```python
from build123d import *

# Parameters (mm, degrees)
SKETCH1_R           = 47.5
SKETCH1_R_2         = 10.5
SKETCH1_R_3         = 2.7
BOSS_EXTRUDE1_DEPTH = 6
SKETCH2_R           = 12
CUT_EXTRUDE1_DEPTH  = 2
BOSS_EXTRUDE2_START = 3
SKETCH3_R           = 16
SKETCH3_R_2         = 12
BOSS_EXTRUDE2_DEPTH = 3
SKETCH4_R           = 2.7
CUT_EXTRUDE2_DEPTH  = 5


with BuildPart() as part:
    # Sketch1 → Boss-Extrude1 (new body)
    with BuildSketch(Plane.XY):
        Circle(SKETCH1_R)
        Circle(SKETCH1_R_2, mode=Mode.SUBTRACT)
        with Locations((44, 0)):
            Circle(SKETCH1_R_3, mode=Mode.SUBTRACT)
        with Locations((22, -38.105117767)):
            Circle(SKETCH1_R_3, mode=Mode.SUBTRACT)
        with Locations((-22, -38.105117767)):
            Circle(SKETCH1_R_3, mode=Mode.SUBTRACT)
        with Locations((-44, 0)):
            Circle(SKETCH1_R_3, mode=Mode.SUBTRACT)
        with Locations((-22, 38.105117767)):
            Circle(SKETCH1_R_3, mode=Mode.SUBTRACT)
        with Locations((22, 38.105117767)):
            Circle(SKETCH1_R_3, mode=Mode.SUBTRACT)
    extrude(amount=BOSS_EXTRUDE1_DEPTH)

    # Sketch2 → Cut-Extrude1 (cut)
    with BuildSketch(Plane(origin=(0, 0, 0), x_dir=(-1, 0, 0), z_dir=(0, 0, -1))):
        Circle(SKETCH2_R)
    extrude(amount=-CUT_EXTRUDE1_DEPTH, mode=Mode.SUBTRACT)

    # Sketch3 → Boss-Extrude2 (add)
    with BuildSketch(Plane(origin=(0, 0, 0), x_dir=(-1, 0, 0), z_dir=(0, 0, -1)).offset(BOSS_EXTRUDE2_START)):
        with Locations(Location((0, 0, 0), (0, 0, 180))):
            Circle(SKETCH3_R)
        Circle(SKETCH3_R_2, mode=Mode.SUBTRACT)
    extrude(amount=-BOSS_EXTRUDE2_DEPTH)

    # Sketch4 → Cut-Extrude2 (cut)
    with BuildSketch(Plane.XY.offset(6)):
        with Locations((8.80698434, 27.105110714)):
            Circle(SKETCH4_R)
        with Locations(Location((-8.80698434, 27.105110714, 0), (0, 0, 180))):
            Circle(SKETCH4_R)
        with Locations(Location((8.80698434, -27.105110714, 0), (0, 0, 180))):
            Circle(SKETCH4_R)
        with Locations((-8.80698434, -27.105110714)):
            Circle(SKETCH4_R)
    extrude(amount=-CUT_EXTRUDE2_DEPTH, mode=Mode.SUBTRACT)


solid = part.part
```
The listing builds one solid part. Answer for the finished solid, in the listing's coordinates (mm). A direction names the side the tool comes from. Coordinates: 2 decimals unless noted, no trailing zeros. Loops run counter-clockwise (first coordinate to the right, second up) from the corner with the lowest first, then second, coordinate; pieces in that order, holes last. Notation, with made-up numbers: (-38.75, 61) -> (13.25, 61) arc R22 ccw to (13.25, 70) -> close; hole circle Ø1 at (-20, 29.25). An arc over 180 degrees is marked (long way). Use one line per item in the form item = value. Start each with the question number.
Item 1: The part is cut by section C-C on z = 4. Count the separate pieces of the cut face and the enclosed holes in it, then the cut area to 3 significant figures.
Item 2: A tool of negligible diameter and unlimited length cuts with its end or side. For faces 5 (the face through (23.25, 35.71, 2.96)), 6 (the face through (11.99, 0.53, -0.54)), 7 (the face through (9, -27, 1)), from which of +Z, -Z, +X, -X, +Y, -Y can it reach the whole face along a straight path? Write none if from no direction.
Item 3: The part is cut by section A-A on y = 0. Determine the outline of the cut face in (x, z).
Item 4: The part is cut by section B-B on x = -44. Determine the outline of the cut face in (y, z).
Item 5: Flat-ended cylindrical pins translate along their axes: pin 1 Ø2.5 at (x, y) = (9.5, 27.5) entering from +Z; pin 2 Ø6 at (x, y) = (-9.5, -27.5) entering from +Z; pin 3 Ø2 at (x, y) = (-22, -16) entering from -Z; pin 4 Ø2 at (y, z) = (-9, 2) entering from -X. Find the tip coordinate at first contact, or state that the pin passes through.
Item 6: The part is cut by section D-D on z = -1.5. Determine the outline of the cut face in (x, y).
Item 7: Consider L1, parallel to Y at x = 22.5, z = 3.5; L2, parallel to X at y = -29, z = 2; L3, parallel to Z at x = -26.5, y = 13.5. Determine where each line is inside the solid, lowest interval first. Write a range as [from, to].
Item 8: The mould has two halves that part along X. Classify faces 1 (the face through (-10.3, -46.37, 2.96)), 2 (the face through (-1, 11, 6)), 3 (the face through (10, 3.2, 4)), 4 (the face through (46.575, 0.811, 2.958)): released by +X, released by -X, zero draft, split by the parting line, or undercut.
Answer key:
q1.separate_pieces = 1
q1.enclosed_holes = 11
q1.area = 6,510 mm2
q2.face_5 = +Z, -Z
q2.face_6 = -Z
q2.face_7 = +Z
q3.outline = (-47.5, 0) -> (-46.7, 0) -> (-46.7, 6) -> (-47.5, 6) -> close; (-41.3, 0) -> (-16, 0) -> (-16, -3) -> (-12, -3) -> (-12, 2) -> (-10.5, 2) -> (-10.5, 6) -> (-41.3, 6) -> close; (10.5, 2) -> (12, 2) -> (12, -3) -> (16, -3) -> (16, 0) -> (41.3, 0) -> (41.3, 6) -> (10.5, 6) -> close; (46.7, 0) -> (47.5, 0) -> (47.5, 6) -> (46.7, 6) -> close
q4.outline = (-17.9, 0) -> (-2.7, 0) -> (-2.7, 6) -> (-17.9, 6) -> close; (2.7, 0) -> (17.9, 0) -> (17.9, 6) -> (2.7, 6) -> close
q5.pin_1 = 1
q5.pin_2 = 6
q5.pin_3 = 0
q5.pin_4 = -46.82
q6.outline = circle Ø32 at (0, 0); hole circle Ø24 at (0, 0)
q7.L1 = [-41.83, -40.76], [-35.45, 35.45], [40.76, 41.83]
q7.L2 = [-37.62, -10.73], [-6.88, 6.88], [10.73, 37.62]
q7.L3 = [0, 6]
q8.face_1 = split by the parting line
q8.face_2 = zero draft
q8.face_3 = undercut
q8.face_4 = undercut
